Could you check a few things on this model? Use its own coordinates, in mm. Round coordinates to 2 decimals unless told otherwise and drop trailing zeros. Write each loop counter-clockwise with the first axis right and the second up, starting at its lowest first coordinate (ties: lowest second). Pieces come first, ordered by that corner, then holes. Notation, with made-up numbers: (-37.75, 7.25) -> (-5.75, 7.25) arc R32 ccw to (-5.75, 40.25) -> close; hole circle Ø9 at (11, 16.5). An arc over 180 degrees is marked (long way). Return JSON: item names as keys, results as strings.
from build123d import *

# Parameters (mm, degrees)
CYLINDER250_R               = 1.5
CYLINDER250_DEPTH           = 20
CYLINDER250_PLACEMENT_ANGLE = 45
CYLINDER251_R               = 1.5
CYLINDER251_DEPTH           = 20
CYLINDER252_R               = 1.5
CYLINDER252_DEPTH           = 20
CYLINDER252_PLACEMENT_ANGLE = 135
CYLINDER247_R               = 1.5
CYLINDER247_DEPTH           = 20
CYLINDER249_R               = 1.5
CYLINDER249_DEPTH           = 20
CYLINDER249_PLACEMENT_ANGLE = 225
CYLINDER246_R               = 1.5
CYLINDER246_DEPTH           = 20
CYLINDER248_R               = 1.5
CYLINDER248_DEPTH           = 20
CYLINDER248_PLACEMENT_ANGLE = 45
CYLINDER245_R               = 1.5
CYLINDER245_DEPTH           = 20
COMPOUND224_PLACEMENT_ANGLE = 22.5
TUBE025_R                   = 52
TUBE025_R_2                 = 42
TUBE025_DEPTH               = 3


with BuildPart() as obj1:
    # Cylinder250 → Cylinder250 (new body)
    with BuildSketch(Plane.XY):
        Circle(CYLINDER250_R)
    extrude(amount=CYLINDER250_DEPTH)


with BuildPart() as obj1_1:
    # Cylinder250 placement: moved
    add(obj1.part.moved(Location((-31.819805, 31.819805, -18))).rotate(Axis((-31.819805, 31.819805, -18), (0, 0, 1)), CYLINDER250_PLACEMENT_ANGLE))


with BuildPart() as obj2:
    # Cylinder251 → Cylinder251 (new body)
    with BuildSketch(Plane(origin=(-45, 0, -18), x_dir=(0, 1, 0), z_dir=(0, 0, 1))):
        Circle(CYLINDER251_R)
    extrude(amount=CYLINDER251_DEPTH)


with BuildPart() as obj3:
    # Cylinder252 → Cylinder252 (new body)
    with BuildSketch(Plane.XY):
        Circle(CYLINDER252_R)
    extrude(amount=CYLINDER252_DEPTH)


with BuildPart() as obj3_1:
    # Cylinder252 placement: moved
    add(obj3.part.moved(Location((-31.819805, -31.819805, -18))).rotate(Axis((-31.819805, -31.819805, -18), (0, 0, 1)), CYLINDER252_PLACEMENT_ANGLE))


with BuildPart() as obj4:
    # Cylinder247 → Cylinder247 (new body)
    with BuildSketch(Plane(origin=(0, -45, -18), x_dir=(-1, 0, 0), z_dir=(0, 0, 1))):
        Circle(CYLINDER247_R)
    extrude(amount=CYLINDER247_DEPTH)


with BuildPart() as obj5:
    # Cylinder249 → Cylinder249 (new body)
    with BuildSketch(Plane.XY):
        Circle(CYLINDER249_R)
    extrude(amount=CYLINDER249_DEPTH)


with BuildPart() as obj5_1:
    # Cylinder249 placement: moved
    add(obj5.part.moved(Location((31.819805, -31.819805, -18))).rotate(Axis((31.819805, -31.819805, -18), (0, 0, 1)), CYLINDER249_PLACEMENT_ANGLE))


with BuildPart() as obj6:
    # Cylinder246 → Cylinder246 (new body)
    with BuildSketch(Plane(origin=(45, 0, -18), x_dir=(0, -1, 0), z_dir=(0, 0, 1))):
        Circle(CYLINDER246_R)
    extrude(amount=CYLINDER246_DEPTH)


with BuildPart() as obj7:
    # Cylinder248 → Cylinder248 (new body)
    with BuildSketch(Plane.XY):
        Circle(CYLINDER248_R)
    extrude(amount=CYLINDER248_DEPTH)


with BuildPart() as obj7_1:
    # Cylinder248 placement: moved
    add(obj7.part.moved(Location((31.819805, 31.819805, -18))).rotate(Axis((31.819805, 31.819805, -18), (0, 0, -1)), CYLINDER248_PLACEMENT_ANGLE))


with BuildPart() as compound224:
    # Cylinder245 → Cylinder245 (new body)
    with BuildSketch(Plane(origin=(0, 45, -18), x_dir=(1, 0, 0), z_dir=(0, 0, 1))):
        Circle(CYLINDER245_R)
    extrude(amount=CYLINDER245_DEPTH)

    # Compound224: union obj1, obj2, obj3, obj4, obj5, obj6, obj7
    add(obj1_1.part)
    add(obj2.part)
    add(obj3_1.part)
    add(obj4.part)
    add(obj5_1.part)
    add(obj6.part)
    add(obj7_1.part)


with BuildPart() as compound224_1:
    # Compound224 placement: moved
    add(compound224.part.rotate(Axis((0, 0, 0), (0, 0, 1)), COMPOUND224_PLACEMENT_ANGLE))


with BuildPart() as j_max_motor_washer:
    # Tube025 → Tube025 (new body)
    with BuildSketch(Plane.XY.offset(-11)):
        Circle(TUBE025_R)
        Circle(TUBE025_R_2, mode=Mode.SUBTRACT)
    extrude(amount=TUBE025_DEPTH)

    # Cut118: cut Compound224
    add(compound224_1.part, mode=Mode.SUBTRACT)


solid = j_max_motor_washer.part
1) Thinking about a two-plate mould opening in X: for faces 1 (the face through (-41.265, -31.641, -9.521)), 2 (the face through (-17.609, -43.023, -9.521)), 3 (the face through (4, 43, -8)), 4 (the face through (40.06, 12.62, -9.52)), which applies, pulls with the +X half, pulls with the -X half, needs draft (parallel to the pull), parting line crosses it, or undercut?
Return value:
{"face 1": "parting line crosses it", "face 2": "undercut", "face 3": "needs draft", "face 4": "undercut"}
2) If I drill on probe 1 along Y at (x, z) = (-18, -10.7); probe 2 along Y at (x, z) = (1, -9.1), over which ranges is the centre line in solid material (lowest first)? Write a range as [from, to].
Return value:
{"probe 1": "[-48.79, -42.86], [-40.29, -37.95], [37.95, 40.29], [42.86, 48.79]", "probe 2": "[-51.99, -41.99], [41.99, 51.99]"}
3) I want a section at A-A, the plane y = 0. Please give me the cut outline in (x, z), and give its area (3 significant figures).
Return value:
{"outline": "(-52, -11) -> (-42, -11) -> (-42, -8) -> (-52, -8) -> close; (42, -11) -> (52, -11) -> (52, -8) -> (42, -8) -> close", "area": "60.0 mm²"}
4) Will these pins go through, and if not, where does the flat tip stop? pin 1 Ø1.8 at (x, y) = (-41.57, 17.22) entering from +Z; pin 2 Ø1 at (y, z) = (-41, -10.5) entering from +X; pin 3 Ø4 at (x, y) = (-17.22, 41.57) entering from -Z; pin 4 Ø1 at (x, z) = (13.5, -9.5) entering from -Y.
Return value:
{"pin 1": "through", "pin 2": "x = 32.62", "pin 3": "z = -11", "pin 4": "y = -50.35"}
5) I want a section at C-C, the plane y = 45.5. Please give me the cut outline in (x, z), and give its area (3 significant figures).
Return value:
{"outline": "(-25.17, -11) -> (25.17, -11) -> (25.17, -8) -> (-25.17, -8) -> close", "area": "151 mm²"}
